Source: CAD feature listing. Evaluate the final solid. Frame: model axes, mm. A direction names the side the tool comes from. Round coordinates to 2 decimals unless told otherwise and drop trailing zeros. Order: outer loops, then holes, each group sorted by start corner. A loop starts at its lowest first (then second) coordinate and runs counter-clockwise, first axis right, second up. Notation, with made-up numbers: M 88,53.5 L 128,53.5 A8 ccw 128,66.5 Z; hole C 3,17 d10. An arc over 180 degrees is marked long. Use one line per item in the form item = value. Start each with the question number.
Q1. Section A-A (y = -63.5). Return the cut outline in (x, z).
Q2. Section D-D (z = 461.5). Return the cut outline in (x, y).
Q3. Reachability of faces 1 (the cylindrical face through (-0.9, -43.99, 172.87)), 2 (the cylindrical face through (-6.883, -30.995, 517.876)), 3 (the cylindrical face through (-6.883, -30.995, 353.864)), 4 (the cylindrical face through (-0.9, -43.99, 389.13)) from +Z, -Z, +X, -X, +Y, -Y: full face, straight path, thin tool, end or side. Return the list, or none.
Q4. Section B-B (z = 36). Return the cut outline in (x, y).
Q5. Material intervals for probe 1 along Z at (x, y) = (24, 6); probe 2 along Z at (x, y) = (-37, 94); probe 3 along Z at (x, y) = (32, 1.5), sorted ascending.
Q6. Pull-direction query (Z, two-part tool) for faces 5 (the flat face through (47.16, 26.07, 98.87)), 6 (the flat face through (-1, 54, 379.5)), 7 (the flat face through (-1, 54, 89.5)); classes: pulls with the +Z half, pulls with the -Z half, needs draft (parallel to the pull), parting line crosses it, or undercut.
Q7. Section C-C (y = -88). Return the cut outline in (x, z).
Q8. Contact query for flat-ended pins moving along their axis: pin 1 (4 mm diameter, centred on x = 19, z = 152, fed in from -Y); pin 2 (6 mm diameter, centred on x = 28.5, y = 23, fed in from +Z); pin 3 (10 mm diameter, centred on x = 2.5, z = 240, fed in from +Y). Output: stop coordinate, or through.
from build123d import *

# Parameters (mm, degrees)
SKETCH1_R           = 31.75
BOSS_EXTRUDE1_DEPTH = 89.5
BOSS_EXTRUDE2_DEPTH = 19
SKETCH3_R           = 38
BOSS_EXTRUDE3_DEPTH = 55
BOSS_EXTRUDE4_DEPTH = 19
SKETCH6_R           = 31.75
BOSS_EXTRUDE5_DEPTH = 52
BOSS_EXTRUDE6_DEPTH = 19
SKETCH8_R           = 38
BOSS_EXTRUDE7_DEPTH = 27.5


with BuildPart() as part:
    # Sketch1 → Boss-Extrude1 (new body)
    with BuildSketch(Plane.XY):
        Circle(SKETCH1_R)
    extrude(amount=BOSS_EXTRUDE1_DEPTH)

    # Sketch2 → Boss-Extrude2 (add)
    with BuildSketch(Plane.XY.offset(89.5)):
        with BuildLine():
            Line((-50.689176209, 57.877952756), (-43.731838298, -4.850393701))
            ThreePointArc((-43.731838298, -4.850393701), (0, -44), (43.731838298, -4.850393701))
            Line((43.731838298, -4.850393701), (50.689176209, 57.877952756))
            ThreePointArc((50.689176209, 57.877952756), (0, 114.5), (-50.689176209, 57.877952756))
        make_face()
    extrude(amount=BOSS_EXTRUDE2_DEPTH)

    # Sketch3 → Boss-Extrude3 (add)
    with BuildSketch(Plane.XY.offset(108.5)):
        with Locations((0, 63.5)):
            Circle(SKETCH3_R)
    extrude(amount=BOSS_EXTRUDE3_DEPTH)

    # Sketch5 → Boss-Extrude4 (add)
    with BuildSketch(Plane.XY.offset(163.5)):
        with BuildLine():
            Line((-50.689176209, 57.877952756), (-43.731838298, -4.850393701))
            ThreePointArc((-43.731838298, -4.850393701), (0, -44), (43.731838298, -4.850393701))
            Line((43.731838298, -4.850393701), (50.689176209, 57.877952756))
            ThreePointArc((50.689176209, 57.877952756), (0, 114.5), (-50.689176209, 57.877952756))
        make_face()
    extrude(amount=BOSS_EXTRUDE4_DEPTH)

    # Sketch6 → Boss-Extrude5 (add)
    with BuildSketch(Plane.XY.offset(182.5)):
        Circle(SKETCH6_R)
    extrude(amount=BOSS_EXTRUDE5_DEPTH)

    # Sketch7 → Boss-Extrude6 (add)
    with BuildSketch(Plane.XY.offset(234.5)):
        with BuildLine():
            Line((50.689176209, -57.877952756), (43.731838298, 4.850393701))
            ThreePointArc((43.731838298, 4.850393701), (0, 44), (-43.731838298, 4.850393701))
            Line((-43.731838298, 4.850393701), (-50.689176209, -57.877952756))
            ThreePointArc((-50.689176209, -57.877952756), (0, -114.5), (50.689176209, -57.877952756))
        make_face()
    extrude(amount=BOSS_EXTRUDE6_DEPTH)

    # Sketch8 → Boss-Extrude7 (add)
    with BuildSketch(Plane.XY.offset(253.5)):
        with Locations((0, -63.5)):
            Circle(SKETCH8_R)
    extrude(amount=BOSS_EXTRUDE7_DEPTH)

    # Mirror3: part across plane


with BuildPart() as part_1:
    add(part.part)
    add(part.part.mirror(Plane.XY.offset(281)))


solid = part_1.part
Results list:
q1.outline = M -51,234.5 L 51,234.5 L 51,253.5 L 38,253.5 L 38,308.5 L 51,308.5 L 51,327.5 L -51,327.5 L -51,308.5 L -38,308.5 L -38,253.5 L -51,253.5 Z
q2.outline = M -50.69,57.88 L -43.73,-4.85 A44 ccw 43.73,-4.85 L 50.69,57.88 A51 ccw long Z
q3.face_1 = -Z, -Y
q3.face_2 = +Z
q3.face_3 = none
q3.face_4 = +Z, -Y
q4.outline = C 0,0 d63.5
q5.probe_1 = 0 to 108.5, 163.5 to 253.5, 308.5 to 398.5, 453.5 to 562
q5.probe_2 = 89.5 to 108.5, 163.5 to 182.5, 379.5 to 398.5, 453.5 to 472.5
q5.probe_3 = 89.5 to 108.5, 163.5 to 182.5, 234.5 to 253.5, 308.5 to 327.5, 379.5 to 398.5, 453.5 to 472.5
q6.face_5 = needs draft
q6.face_6 = undercut
q6.face_7 = pulls with the -Z half
q7.outline = M -44.73,234.5 L 44.73,234.5 L 44.73,253.5 L 29.05,253.5 L 29.05,308.5 L 44.73,308.5 L 44.73,327.5 L -44.73,327.5 L -44.73,308.5 L -29.05,308.5 L -29.05,253.5 L -44.73,253.5 Z
q8.pin_1 = 29.51
q8.pin_2 = 472.5
q8.pin_3 = 44
